The drawing under review shows one solid part. Ordinate dimensions are in mm from its lowest x, y, z. Coordinates: 2 decimals unless noted, no trailing zeros. Write each loop counter-clockwise with the first axis right and the second up, starting at its lowest first coordinate (ties: lowest second). Pieces come first, ordered by that corner, then holes. Notation, with made-up numbers: (-20, 15) - (7, 15) arc R23 cw to (7, 51) - close; hole circle Ø2 at (40, 24.25). An arc over 180 degrees is marked (long way). Put each result on its own line as item: value. Start each with the question number.
Item 1: Consider section A-A on y = 30. Give the boundary of the cut face in (x, z) (1 decimal).
Item 2: Consider section C-C on z = 1.95. State how many separate pieces and enclosed holes the cut face has, then the cut area to 3 significant figures.
Item 3: Consider section D-D on x = 44.5. Give the boundary of the cut face in (y, z).
Item 4: To check wall thickness, follow L1, parallel to Y at x = 30, z = 1.6 (1 decimal); L2, parallel to X at y = 31, z = 2.1 (1 decimal); L3, parallel to X at y = 5, z = 1.15 (1 decimal). State the ranges of each line that lie inside material, in increasing order. Write a range as [from, to].
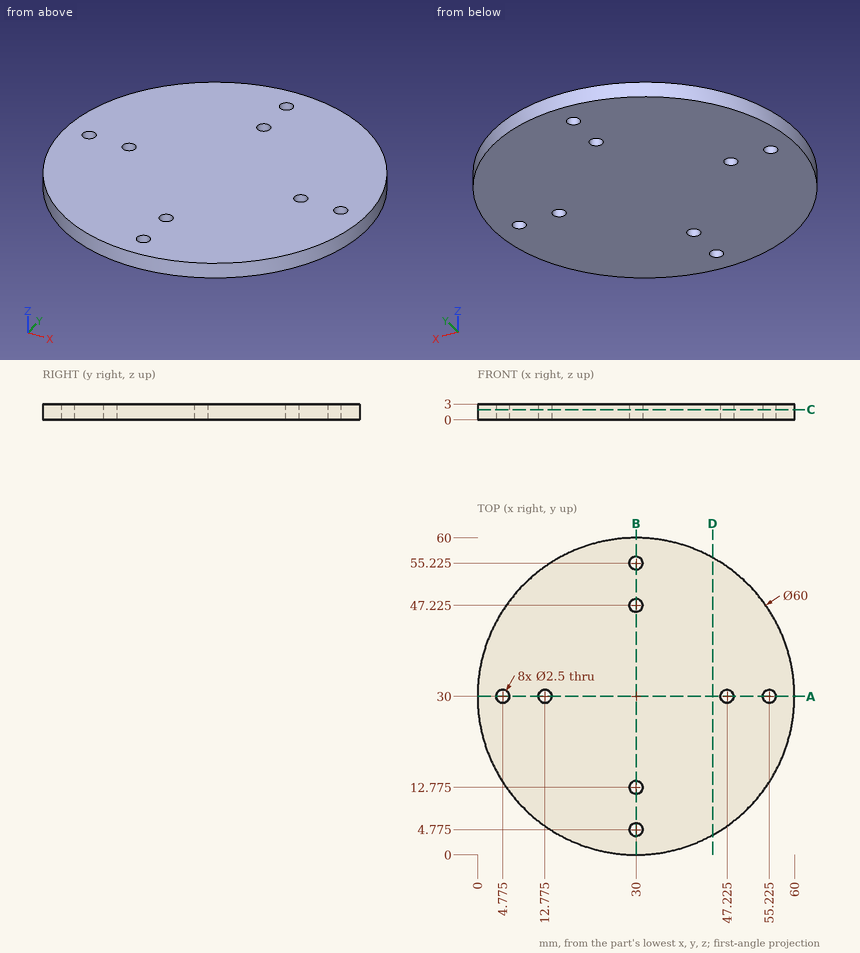
Report:
1. outline: (0, 0) - (3.5, 0) - (3.5, 3) - (0, 3) - close; (6, 0) - (11.5, 0) - (11.5, 3) - (6, 3) - close; (14, 0) - (46, 0) - (46, 3) - (14, 3) - close; (48.5, 0) - (54, 0) - (54, 3) - (48.5, 3) - close; (56.5, 0) - (60, 0) - (60, 3) - (56.5, 3) - close
2. separate pieces: 1
2. enclosed holes: 8
2. area: 2,790 mm²
3. outline: (3.74, 0) - (56.26, 0) - (56.26, 3) - (3.74, 3) - close
4. L1: [0, 3.5], [6, 11.5], [14, 46], [48.5, 54], [56.5, 60]
4. L2: [0, 4], [5.5, 12], [13.5, 46.5], [48, 54.5], [56, 60]
4. L3: [13.4, 28.8], [31.2, 46.6]
